from build123d import *
from build123d.topology import SkipClean

# Parameters (mm, degrees)
BOSS_EXTRU_1_DEPTH      = 2.5
ESQUISSE2_W             = 5
ESQUISSE2_H             = 8
BOSS_EXTRU_2_DEPTH      = 22
ENL_V_MAT_EXTRU_2_REACH = 71.856
ESQUISSE4_R             = 1.6
EXTRU_MINCE1_OUTLINE_W  = 15
EXTRU_MINCE1_OUTLINE_H  = 8
EXTRU_MINCE1_DEPTH      = 19.5
BOSS_EXTRU_3_DEPTH      = 1.3
ESQUISSE3_R             = 2.1
ESQUISSE3_W             = 5
ESQUISSE3_H             = 1.5
ENL_V_MAT_EXTRU_1_DEPTH = 70.856137884
ENL_V_MAT_EXTRU_3_REACH = 76.889
ESQUISSE7_R             = 1.6
ESQUISSE8_W             = 20
ESQUISSE8_H             = 5
ENL_V_MAT_EXTRU_5_DEPTH = 1


# Read off the part's stored shape, not the designer's step: Extru.-Mince1
with BuildPart() as part:
    # Esquisse1 → Boss.-Extru.1 (new body)
    with BuildSketch(Plane(origin=(0, 0, 0), x_dir=(1, 0, 0), z_dir=(0, 1, 0))):
        Polygon((0, 0), (29.2, 0), (29.2, 8), (7, 8), (7, 48.8), (29.2, 48.8), (29.2, 56.8), (0, 56.8), align=None)
    extrude(amount=BOSS_EXTRU_1_DEPTH)

    # Esquisse2 → Boss.-Extru.2 (add)
    with BuildSketch(Plane(origin=(0, 0, 0), x_dir=(1, 0, 0), z_dir=(0, 1, 0))):
        with Locations((31.7, 52.8)):
            Rectangle(ESQUISSE2_W, ESQUISSE2_H)
        with Locations((31.7, 4)):
            Rectangle(ESQUISSE2_W, ESQUISSE2_H)
    extrude(amount=BOSS_EXTRU_2_DEPTH)

    # Esquisse4 → Enlèv. mat.-Extru.2 (cut, up to next)
    with BuildSketch(Plane(origin=(0, 0, 0), x_dir=(1, 0, 0), z_dir=(0, 1, 0)), mode=Mode.PRIVATE) as enl_v_mat_extru_2_sk1:
        with Locations(Location((3.5, 14.4, 0), (0, 0, 270))):
            Circle(ESQUISSE4_R)
    enl_v_mat_extru_2_tool1 = extrude(enl_v_mat_extru_2_sk1.sketch, amount=ENL_V_MAT_EXTRU_2_REACH, mode=Mode.PRIVATE) & part.part
    # Esquisse4 → Enlèv. mat.-Extru.2 (cut, up to next)
    with BuildSketch(Plane(origin=(0, 0, 0), x_dir=(1, 0, 0), z_dir=(0, 1, 0)), mode=Mode.PRIVATE) as enl_v_mat_extru_2_sk2:
        with Locations(Location((3.5, 42.4, 0), (0, 0, 90))):
            Circle(ESQUISSE4_R)
    enl_v_mat_extru_2_tool2 = extrude(enl_v_mat_extru_2_sk2.sketch, amount=ENL_V_MAT_EXTRU_2_REACH, mode=Mode.PRIVATE) & part.part
    add(enl_v_mat_extru_2_tool1.solids().sort_by_distance((3.5, 0, -14.4))[0], mode=Mode.SUBTRACT)
    add(enl_v_mat_extru_2_tool2.solids().sort_by_distance((3.5, 0, -42.4))[0], mode=Mode.SUBTRACT)

    # Extru.-Mince1 outline → Extru.-Mince1 (add)
    with BuildSketch(Plane(origin=(0, 2.5, 0), x_dir=(1, 0, 0), z_dir=(0, 1, 0))):
        with Locations((21.7, 52.8)):
            Rectangle(EXTRU_MINCE1_OUTLINE_W, EXTRU_MINCE1_OUTLINE_H)
        Polygon((27.7, 50.3), (20.2, 50.3), (27.7, 54.3), align=None, mode=Mode.SUBTRACT)
        Polygon((15.7, 51.3), (15.7, 55.3), (23.2, 55.3), align=None, mode=Mode.SUBTRACT)
    extru_mince1 = extrude(amount=EXTRU_MINCE1_DEPTH)

    # Esquisse6 → Boss.-Extru.3 (add)
    with BuildSketch(Plane.XZ):
        Polygon((34.2, -8), (7, -8), (7, -48.8), (34.2, -48.8), (34.2, -56.8), (44.2, -56.8), (44.2, 0), (34.2, 0), align=None)
    extrude(amount=-BOSS_EXTRU_3_DEPTH)

    # Esquisse3 → Enlèv. mat.-Extru.1 (cut, through all)
    with BuildSketch(Plane(origin=(34.2, 0, 0), x_dir=(0, 0, -1), z_dir=(1, 0, 0))):
        with Locations((3.8, 6.1)):
            Circle(ESQUISSE3_R)
        with Locations((53, 6.1)):
            Circle(ESQUISSE3_R)
        with Locations((3.8, 16.85)):
            Rectangle(ESQUISSE3_W, ESQUISSE3_H)
        with Locations((53, 16.85)):
            Rectangle(ESQUISSE3_W, ESQUISSE3_H)
    enl_v_mat_extru_1 = extrude(amount=-ENL_V_MAT_EXTRU_1_DEPTH, mode=Mode.SUBTRACT)

    # Symétrie1: Extru.-Mince1, Enlèv. mat.-Extru.1 across plane
    with SkipClean():  # the faces are left unmerged after this step: merging them gives an invalid solid
        add(extru_mince1.mirror(Plane(origin=(0, 0, -28.4), x_dir=(1, 0, 0), z_dir=(0, 0, -1))))
        add(enl_v_mat_extru_1.mirror(Plane(origin=(0, 0, -28.4), x_dir=(1, 0, 0), z_dir=(0, 0, -1))), mode=Mode.SUBTRACT)

    # Esquisse7 → Enlèv. mat.-Extru.3 (cut, up to next)
    with BuildSketch(Plane(origin=(0, 1.3, 0), x_dir=(1, 0, 0), z_dir=(0, 1, 0)), mode=Mode.PRIVATE) as enl_v_mat_extru_3_sk1:
        with Locations(Location((39.2, 52.8, 0), (0, 0, 270))):
            Circle(ESQUISSE7_R)
    enl_v_mat_extru_3_tool1 = extrude(enl_v_mat_extru_3_sk1.sketch, amount=-ENL_V_MAT_EXTRU_3_REACH, mode=Mode.PRIVATE) & part.part
    # Esquisse7 → Enlèv. mat.-Extru.3 (cut, up to next)
    with BuildSketch(Plane(origin=(0, 1.3, 0), x_dir=(1, 0, 0), z_dir=(0, 1, 0)), mode=Mode.PRIVATE) as enl_v_mat_extru_3_sk2:
        with Locations(Location((39.2, 4, 0), (0, 0, 270))):
            Circle(ESQUISSE7_R)
    enl_v_mat_extru_3_tool2 = extrude(enl_v_mat_extru_3_sk2.sketch, amount=-ENL_V_MAT_EXTRU_3_REACH, mode=Mode.PRIVATE) & part.part
    add(enl_v_mat_extru_3_tool1.solids().sort_by_distance((39.2, 1.3, -52.8))[0], mode=Mode.SUBTRACT)
    add(enl_v_mat_extru_3_tool2.solids().sort_by_distance((39.2, 1.3, -4))[0], mode=Mode.SUBTRACT)

    # Esquisse8 → Enlèv. mat.-Extru.5 (cut)
    with SkipClean():  # the faces are left unmerged after this step: merging them gives an invalid solid
        with BuildSketch(Plane(origin=(0, 22, 0), x_dir=(1, 0, 0), z_dir=(0, 1, 0))):
            with Locations((24.2, 52.8)):
                Rectangle(ESQUISSE8_W, ESQUISSE8_H)
            with Locations((24.2, 4)):
                Rectangle(ESQUISSE8_W, ESQUISSE8_H)
        extrude(amount=-ENL_V_MAT_EXTRU_5_DEPTH, mode=Mode.SUBTRACT)


solid = part.part
The listing builds one solid part. Answer for the finished solid, in the listing's coordinates (mm). A direction names the side the tool comes from. Coordinates: 2 decimals unless noted, no trailing zeros. Loops run counter-clockwise (first coordinate to the right, second up) from the corner with the lowest first, then second, coordinate; pieces in that order, holes last. Notation, with made-up numbers: (78.5, 83) -> (127.5, 83) arc R17 cw to (127.5, 87) -> close; hole circle Ø2 at (-15, 67). An arc over 180 degrees is marked (long way). Answer in a Markdown table with one row per item. Add a question column.
1. Flat-ended cylindrical pins translate along their axes: P1, Ø4, axis at y = 16.5, z = -53, coming from the -X side; P2, Ø1.3, axis at y = 2, z = -36, coming from the +X side; P3, Ø7, axis at x = 5.5, z = -16.5, coming from the +Y side; P4, Ø1.9, axis at x = 3.5, z = -42.4, coming from the -Y side. Find the tip coordinate at first contact, or state that the pin passes through.
2. Determine the mould class of faces 1 (the flat face through (23, 12, -8)), 2 (the flat face through (14.2, 12, -4)), 3 (the flat face through (19, 2.5, -54)) for opening direction X: +X half, -X half, draft (parallel to the pull), parting line (faces both ways), or undercut.
3. The part is cut by section B-B, the plane x = 3.5. Write down the section's boundary in (y, z).
4. Consider line 1 (Y direction, x = 20.5, z = -3.8); line 2 (Z direction, x = 30.5, y = 16.25); line 3 (X direction, y = 0.7, z = -4). Determine where each line is inside the solid, lowest interval first. Write a range as [from, to].
5. The part is cut by section A-A, the plane y = 14.5. Write down the section's boundary in (x, z).
6. For faces 4 (the flat face through (26, 2.5, -51)), 5 (the flat face through (5, 2.5, -29)), 6 (the flat face through (24, 22, -1)), 7 (the flat face through (24, 16.1, -53)), determine the directions among +Z, -Z, +X, -X, +Y, -Y from which every point of the face is accessible in a straight line to the end or side of a thin tool.
7. The part is cut by section C-C, the plane z = -14.4. Write down the section's boundary in (x, y), then the cut area to 3 significant figures.
8. The part is cut by section D-D, the plane x = 39.2. Write down the section's boundary in (y, z), then the cut area to 3 significant figures.
Answer below:
| question | item | result |
|---|---|---|
| 1 | P1 | x = 14.2 |
| 1 | P2 | x = 7 |
| 1 | P3 | y = 2.5 |
| 1 | P4 | through |
| 2 | face 1 | draft |
| 2 | face 2 | -X half |
| 2 | face 3 | undercut |
| 3 | outline | (0, -56.8) -> (2.5, -56.8) -> (2.5, -44) -> (0, -44) -> close; (0, -40.8) -> (2.5, -40.8) -> (2.5, -16) -> (0, -16) -> close; (0, -12.8) -> (2.5, -12.8) -> (2.5, 0) -> (0, 0) -> close |
| 4 | line 1 | [0, 4], [8.2, 16.1], [17.6, 21] |
| 4 | line 2 | [-56.8, -55.5], [-50.5, -48.8], [-8, -6.3], [-1.3, 0] |
| 4 | line 3 | [0, 37.6], [40.8, 44.2] |
| 5 | outline | (14.2, -56.8) -> (34.2, -56.8) -> (34.2, -48.8) -> (14.2, -48.8) -> close; (14.2, -8) -> (34.2, -8) -> (34.2, 0) -> (14.2, 0) -> close; hole (15.7, -55.3) -> (23.2, -55.3) -> (15.7, -51.3) -> close; hole (15.7, -5.5) -> (23.2, -1.5) -> (15.7, -1.5) -> close; hole (20.2, -50.3) -> (27.7, -54.3) -> (27.7, -50.3) -> close; hole (20.2, -6.5) -> (27.7, -6.5) -> (27.7, -2.5) -> close |
| 6 | face 4 | +Y |
| 6 | face 5 | +Z, -Z, -X, +Y |
| 6 | face 6 | +Z, -Z, +X, -X, +Y |
| 6 | face 7 | +X, -X |
| 7 | outline | (0, 0) -> (1.9, 0) -> (1.9, 2.5) -> (0, 2.5) -> close; (5.1, 0) -> (44.2, 0) -> (44.2, 1.3) -> (7, 1.3) -> (7, 2.5) -> (5.1, 2.5) -> close |
| 7 | area | 57.9 mm2 |
| 8 | outline | (0, -56.8) -> (1.3, -56.8) -> (1.3, -54.4) -> (0, -54.4) -> close; (0, -51.2) -> (1.3, -51.2) -> (1.3, -5.6) -> (0, -5.6) -> close; (0, -2.4) -> (1.3, -2.4) -> (1.3, 0) -> (0, 0) -> close |
| 8 | area | 65.5 mm2 |
